For this review, take the finished solid that the model builds, in its own axes (mm). A direction names the side the tool comes from. Coordinates: 2 decimals unless noted, no trailing zeros. Loops run counter-clockwise (first coordinate to the right, second up) from the corner with the lowest first, then second, coordinate; pieces in that order, holes last. Notation, with made-up numbers: (-12, 22) - (0, 22) arc R7 ccw to (0, 30) - close; hole circle Ø6 at (4.5, 33.25). An arc over 180 degrees is marked (long way). One line per item, written item: value. Start each with the question number.
1. To check wall thickness, follow line 1 (X direction, y = -34, z = -4); line 2 (Z direction, x = 48.15, y = 43). State the ranges of each line that lie inside material, in increasing order. Write a range as from..to.
2. Insertion check: pin 1 (3.5 mm diameter, centred on y = 43, z = -5, fed in from -X); pin 2 (2.5 mm diameter, centred on x = -43, z = -5, fed in from +Y); pin 3 (2.5 mm diameter, centred on x = -42.5, z = -5, fed in from -Y). Each pin has a flat end and moves straight along its axis. Give the tip position at first contact, or say it passes through.
3. Take a section at A-A, the plane y = 35. Count the separate pieces of the cut face and the enclosed holes in it, and give its area (3 significant figures).
4. Take a section at B-B, the plane x = -28.5. State the section outline as (y, z) points, and give its area (3 significant figures).
5. The part is to be moulded in two halves that separate along Y. For faces 1 (the face through (15, 44, -5)), 2 (the face through (-40.92, -47.04, -5.86)), 3 (the face through (12, 37, -8)), say which applies: released by +Y, released by -Y, zero draft, split by the parting line, or undercut.
6. For faces 4 (the face through (-19, 31, -6)), 5 (the face through (-1, -40, -5)), 6 (the face through (47.04, -40.92, -5.86)), 7 (the face through (-47.04, 40.92, -5.86)), list the 3-axis set-ups (+Z, -Z, +X, -X, +Y, -Y) from which the entire face can be reached by the end or side of a thin tool; tool diameter is ignored.
```python
from build123d import *

# Parameters (mm, degrees)
SKETCH081_W           = 100
SKETCH081_H           = 100
SKETCH081_W_2         = 80
SKETCH081_H_2         = 80
PAD032_DEPTH          = 10
SKETCH083_R           = 2.25
POCKET051_DEPTH       = 6
POLARPATTERN002_COUNT = 4
SKETCH082_R           = 2.25
POCKET050_DEPTH       = 6
POLARPATTERN003_COUNT = 4
SKETCH084_R           = 2.25
POCKET049_DEPTH       = 6
SKETCH098_R           = 2.2
PAD037_DEPTH          = 4
POCKET061_DEPTH       = 2.5


with BuildPart() as part:
    # Sketch081 → Pad032 (new body)
    with BuildSketch(Plane.XY):
        Rectangle(SKETCH081_W, SKETCH081_H)
        Rectangle(SKETCH081_W_2, SKETCH081_H_2, mode=Mode.SUBTRACT)
    extrude(amount=PAD032_DEPTH)

    # Sketch083 → Pocket051 (cut)
    with BuildSketch(Plane.XZ.offset(50)):
        with Locations((-43, 5)):
            Circle(SKETCH083_R)
    pocket051 = extrude(amount=-POCKET051_DEPTH, mode=Mode.SUBTRACT)

    # PolarPattern002: Pocket051 ×4 about axis
    polarpattern002_axis = Axis((0, 0, 0), (0, 0, 1))
    for i in range(1, POLARPATTERN002_COUNT):
        add(pocket051.rotate(polarpattern002_axis, i * 360 / POLARPATTERN002_COUNT), mode=Mode.SUBTRACT)

    # Sketch082 (on Face2 of PolarPattern002) → Pocket050 (cut)
    with BuildSketch(Plane(origin=(-50, 0, 0), x_dir=(0, -1, 0), z_dir=(-1, 0, 0))):
        with Locations((43, 5)):
            Circle(SKETCH082_R)
    pocket050 = extrude(amount=-POCKET050_DEPTH, mode=Mode.SUBTRACT)

    # PolarPattern003: Pocket050 ×4 about axis
    polarpattern003_axis = Axis((0, 0, 0), (0, 0, 1))
    for i in range(1, POLARPATTERN003_COUNT):
        add(pocket050.rotate(polarpattern003_axis, i * 360 / POLARPATTERN003_COUNT), mode=Mode.SUBTRACT)

    # Sketch084 (on Face1 of PolarPattern003) → Pocket049 (cut)
    with BuildSketch(Plane(origin=(0, 50, 0), x_dir=(-1, 0, 0), z_dir=(0, 1, 0))):
        with Locations((-15, 5)):
            Circle(SKETCH084_R)
    pocket049 = extrude(amount=-POCKET049_DEPTH, mode=Mode.SUBTRACT)

    # Mirrored003: Pocket049 across Sketch084 V_Axis
    add(pocket049.mirror(Plane(origin=(0, 50, 0), x_dir=(0, 1, 0), z_dir=(-1, 0, 0))), mode=Mode.SUBTRACT)

    # Sketch098 (on Face3 of Mirrored003) → Pad037 (join)
    with BuildSketch(Plane(origin=(0, 0, 0), x_dir=(1, 0, 0), z_dir=(0, 0, -1))):
        with BuildLine():
            Line((-23, -40), (-23, -33.5))
            ThreePointArc((-12, -33.5), (-17.5, -28), (-23, -33.5))
            Line((-12, -40), (-12, -33.5))
            Line((-23, -40), (-12, -40))
        make_face()
        with Locations((-17.5, -35)):
            Circle(SKETCH098_R, mode=Mode.SUBTRACT)
    pad037 = extrude(amount=-PAD037_DEPTH)

    # Sketch099 (on Face29 of Pad037) → Pocket061 (cut)
    with BuildSketch(Plane.XY.offset(4)):
        Polygon((-14, 37.020726), (-17.5, 39.041452), (-21, 37.020726), (-21, 32.979274), (-17.5, 30.958548), (-14, 32.979274), align=None)
    pocket061 = extrude(amount=-POCKET061_DEPTH, mode=Mode.SUBTRACT)

    # Mirrored006: Pad037, Pocket061 across Sketch098 V_Axis
    add(pad037.mirror(Plane(origin=(0, 0, 0), x_dir=(0, 0, -1), z_dir=(1, 0, 0))))
    add(pocket061.mirror(Plane(origin=(0, 0, 0), x_dir=(0, 0, -1), z_dir=(1, 0, 0))), mode=Mode.SUBTRACT)


with BuildPart() as part_1:
    # Body011 placement: moved
    add(part.part.moved(Location((0, 0, -10))))


solid = part_1.part
```
Solutions:
1. line 1: -50..-40, 40..50
1. line 2: -10..-7.25, -2.75..0
2. pin 1: x = -44
2. pin 2: y = 44
2. pin 3: y = -44
3. separate pieces: 6
3. enclosed holes: 0
3. area: 240 mm2
4. outline: (-50, -10) - (-40, -10) - (-40, 0) - (-50, 0) - close; (40, -10) - (50, -10) - (50, 0) - (40, 0) - close
4. area: 200 mm2
5. face 1: released by +Y
5. face 2: zero draft
5. face 3: undercut
6. face 4: +Z
6. face 5: +Z, -Z
6. face 6: +X
6. face 7: -X
